Autodesk Inventor part; units mm, degrees
ref_plane "YZ Plane" through (0, 0, 0) normal (1, 0, 0) x (0, 1, 0)
ref_plane "XZ Plane" through (0, 0, 0) normal (0, 1, 0) x (-1, 0, 0)
ref_plane "XY Plane" through (0, 0, 0) normal (0, 0, 1) x (1, 0, 0)
sketch "Sketch1" plane through (0, 0, 0) normal (1, 0, 0) x (0, 1, 0)
  line L0 (0, 0) -> (0, 25.4)
  line L1 (0, 25.4) -> (11.1252, 25.4)
  line L2 (11.1252, 25.4) -> (11.1252, 5.1054)
  line L3 (11.1252, 5.1054) -> (14.097, 5.1054)
  line L4 (14.097, 5.1054) -> (14.097, 2.54)
  line L5 (14.097, 2.54) -> (6.35, 2.54)
  line L6 (6.35, 2.54) -> (6.35, 0)
  line L7 (6.35, 0) -> (0, 0)
  dimension "d1" = 11.1252
  dimension "d2" = 50.8
  dimension "d3" = 14.097
  dimension "d4" = 5.08
  dimension "d5" = 10.2108
  dimension "d6" = 6.35
revolve "Revolution1" add sketch "Sketch1" angle 360 about axis through (0, 6.35, 0) along (0, -1, 0)
fillet "Fillet1" radius 0.7937 1 edges at (0, 11.1252, -25.4)
properties part number "BIG-MAGNET" material "Steel, Alloy"
Verification items for the finished model (mm, model axes). A direction names the side the tool comes from. Give positions to 0.01 mm unless a question says otherwise; leave off trailing zeros. Loops run counter-clockwise (first coordinate to the right, second up) from the corner with the lowest first, then second, coordinate; pieces in that order, holes last.
1. Tool access check on faces 1 (the cylindrical face through (1.53, 12.63, 4.87)), 2 (the flat face through (2, 14.097, 2)). Record the directions out of +Z, -Z, +X, -X, +Y, -Y that give a thin tool (end or side, any length) a straight path to the whole face; none if there is none.
Derived:
face 1: +Y
face 2: +Z, -Z, +X, -X, +Y
2. Cross-section at B-B on y = 7. Record the cut outline in (x, z), and give its area (3 significant figures).
Derived:
outline: circle Ø50.8 at (0, 0); hole circle Ø5.08 at (0, 0)
area: 2,010 mm2
3. Material ranges on probe 1 along X at (y, z) = (9.25, 0); probe 2 along Z at (x, y) = (0, 12.25), recorded low to high.
Derived:
probe 1: x = -25.4 to -2.54, 2.54 to 25.4
probe 2: z = -5.11 to -2.54, 2.54 to 5.11
4. Go/stop test with flat-tipped pins: P1, Ø8, axis at x = -3.5, z = -8, coming from the +Y side; P2, Ø1, axis at x = -9.5, z = 13, coming from the +Y side; P3, Ø2, axis at y = 11, z = 15, coming from the +X side; P4, Ø4.5, axis at x = 0, z = 0, coming from the +Y side. Record where each tip stops, or that it passes through.
Derived:
P1: stops at y = 14.1
P2: stops at y = 11.13
P3: stops at x = 21.09
P4: stops at y = 6.35
5. Release check for a two-part mould opening along Z. For faces 3 (the flat face through (0, 0, 0)), 4 (the cylindrical face through (-24.796, 5.238, -5.506)), 5 (the flat face through (0, 6.35, 0)) record: +Z half, -Z half, draft (parallel to the pull), parting line (faces both ways), or undercut.
Derived:
face 3: draft
face 4: parting line
face 5: undercut
6. Cross-section at D-D on y = 3.5. Record the cut outline in (x, z).
Derived:
outline: circle Ø50.8 at (0, 0)
7. Cross-section at C-C on x = 0. Record the cut outline in (y, z), and give its area (3 significant figures).
Derived:
outline: (0, -25.4) - (10.33, -25.4) arc R0.79 ccw to (11.13, -24.61) - (11.13, -5.11) - (14.1, -5.11) - (14.1, -2.54) - (6.35, -2.54) - (6.35, 2.54) - (14.1, 2.54) - (14.1, 5.11) - (11.13, 5.11) - (11.13, 24.61) arc R0.79 ccw to (10.33, 25.4) - (0, 25.4) - close
area: 556 mm2
8. Cross-section at A-A on z = 0. Record the cut outline in (x, y), and give its area (3 significant figures).
Derived:
outline: (-25.4, 0) - (25.4, 0) - (25.4, 10.33) arc R0.79 ccw to (24.61, 11.13) - (5.11, 11.13) - (5.11, 14.1) - (2.54, 14.1) - (2.54, 6.35) - (-2.54, 6.35) - (-2.54, 14.1) - (-5.11, 14.1) - (-5.11, 11.13) - (-24.61, 11.13) arc R0.79 ccw to (-25.4, 10.33) - close
area: 556 mm2
